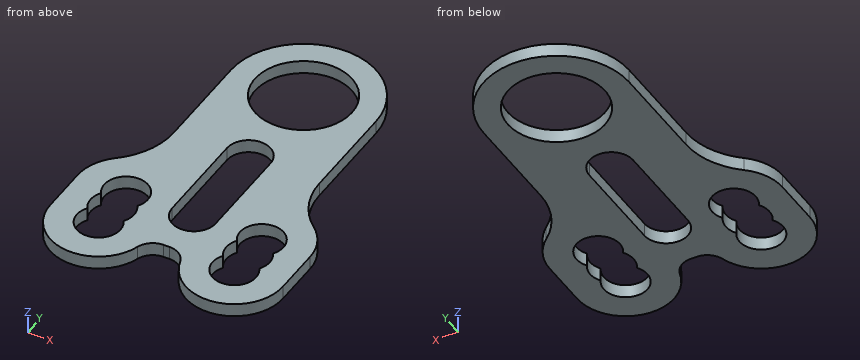
```python
from build123d import *

# Parameters (mm, degrees)
SKETCH_1_R      = 10
EXTRUDE_1_DEPTH = 2.75


with BuildPart() as part:
    # 草图1 → 凸台-拉伸1 (new body)
    with BuildSketch(Plane.XY):
        with BuildLine():
            Line((-24, -40), (-24, -50))
            ThreePointArc((-24, -50), (-15.443695821, -59.895238369), (-4.416851525, -52.857142857))
            ThreePointArc((-4.416851525, -52.857142857), (-2.974049354, -50.792865097), (-0.583592135, -50))
            Line((-0.583592135, -50), (0.583592135, -50))
            ThreePointArc((0.583592135, -50), (2.974049354, -50.792865097), (4.416851525, -52.857142857))
            ThreePointArc((4.416851525, -52.857142857), (15.443695821, -59.895238369), (24, -50))
            Line((24, -50), (24, -40))
            ThreePointArc((24, -40), (23.055385138, -35.757359313), (20.4, -32.316250915))
            ThreePointArc((20.4, -32.316250915), (16.416922293, -27.154588318), (15, -20.790627288))
            Line((15, -20.790627288), (15, 0))
            ThreePointArc((15, 0), (0, 15), (-15, 0))
            Line((-15, 0), (-15, -20.790627288))
            ThreePointArc((-15, -20.790627288), (-16.416922293, -27.154588318), (-20.4, -32.316250915))
            ThreePointArc((-20.4, -32.316250915), (-23.055385138, -35.757359313), (-24, -40))
        make_face()
        Circle(SKETCH_1_R, mode=Mode.SUBTRACT)
        with BuildLine():
            Line((-4.5, -20), (-4.5, -40))
            ThreePointArc((-4.5, -40), (0, -44.5), (4.5, -40))
            Line((4.5, -40), (4.5, -20))
            ThreePointArc((4.5, -20), (0, -15.5), (-4.5, -20))
        make_face(mode=Mode.SUBTRACT)
        with BuildLine():
            ThreePointArc((-17.741657387, -47.5), (-14, -54.5), (-10.258342613, -47.5))
            ThreePointArc((-10.258342613, -47.5), (-9.5, -45), (-10.258342613, -42.5))
            ThreePointArc((-10.258342613, -42.5), (-14, -35.5), (-17.741657387, -42.5))
            ThreePointArc((-17.741657387, -42.5), (-18.5, -45), (-17.741657387, -47.5))
        make_face(mode=Mode.SUBTRACT)
        with BuildLine():
            ThreePointArc((10.258342613, -47.5), (9.5, -45), (10.258342613, -42.5))
            ThreePointArc((10.258342613, -42.5), (14, -35.5), (17.741657387, -42.5))
            ThreePointArc((17.741657387, -42.5), (18.5, -45), (17.741657387, -47.5))
            ThreePointArc((17.741657387, -47.5), (14, -54.5), (10.258342613, -47.5))
        make_face(mode=Mode.SUBTRACT)
    extrude(amount=EXTRUDE_1_DEPTH)


solid = part.part
```
Work out the finished part from the listing and answer in its coordinate system (mm). Give positions to 0.01 mm unless a question says otherwise; leave off trailing zeros. Write each loop counter-clockwise with the first axis right and the second up, starting at its lowest first coordinate (ties: lowest second). Pieces come first, ordered by that corner, then holes. Notation, with made-up numbers: (79, 64) - (89, 64) arc R18 ccw to (89, 81) - close; hole circle Ø5 at (-31.75, 74). An arc over 180 degrees is marked (long way). Use one line per item in the form item = value.
1. A cutting plane is placed at A-A (y = -8). Write down the section's boundary in (x, z).
Filled in:
outline = (-15, 0) - (-6, 0) - (-6, 2.75) - (-15, 2.75) - close; (6, 0) - (15, 0) - (15, 2.75) - (6, 2.75) - close
2. A cutting plane is placed at D-D (y = -46). Write down the section's boundary in (x, z).
Filled in:
outline = (-24, 0) - (-18.39, 0) - (-18.39, 2.75) - (-24, 2.75) - close; (-9.61, 0) - (9.61, 0) - (9.61, 2.75) - (-9.61, 2.75) - close; (18.39, 0) - (24, 0) - (24, 2.75) - (18.39, 2.75) - close
3. Each of these flat-tipped pins is pushed along its axis until it touches: pin 1 Ø1 at (y, z) = (-6.5, 0.5) entering from -X; pin 2 Ø1.4 at (y, z) = (-26.5, 2) entering from -X; pin 3 Ø12 at (x, y) = (2, -34.5) entering from +Z; pin 4 Ø8 at (x, y) = (14, -40) entering from +Z. Where does it stop, or does it pass through?
Filled in:
pin_1 = -15
pin_2 = -16.44
pin_3 = 2.75
pin_4 = through
4. A cutting plane is placed at B-B (z = 1.15). Write down the section's boundary in (x, y), and give its area (3 significant figures).
Filled in:
outline = (-24, -50) arc R10 ccw to (-4.42, -52.86) arc R4 cw to (-0.58, -50) - (0.58, -50) arc R4 cw to (4.42, -52.86) arc R10 ccw to (24, -50) - (24, -40) arc R10 ccw to (20.4, -32.32) arc R15 cw to (15, -20.79) - (15, 0) arc R15 ccw to (-15, 0) - (-15, -20.79) arc R15 cw to (-20.4, -32.32) arc R10 ccw to (-24, -40) - close; hole (-17.74, -47.5) arc R4.5 ccw (long way) to (-10.26, -47.5) arc R4.5 ccw to (-10.26, -42.5) arc R4.5 ccw (long way) to (-17.74, -42.5) arc R4.5 ccw to start; hole circle Ø20 at (0, 0); hole (-4.5, -40) arc R4.5 ccw to (4.5, -40) - (4.5, -20) arc R4.5 ccw to (-4.5, -20) - close; hole (10.26, -47.5) arc R4.5 ccw (long way) to (17.74, -47.5) arc R4.5 ccw to (17.74, -42.5) arc R4.5 ccw (long way) to (10.26, -42.5) arc R4.5 ccw to start
area = 1,660 mm^2
5. A cutting plane is placed at C-C (x = 14). Write down the section's boundary in (y, z).
Filled in:
outline = (-60, 0) - (-54.5, 0) - (-54.5, 2.75) - (-60, 2.75) - close; (-35.5, 0) - (5.39, 0) - (5.39, 2.75) - (-35.5, 2.75) - close
6. Consider L1, parallel to X at y = -40, z = 1.2; L2, parallel to Y at x = 3, z = 1.1; L3, parallel to X at y = -36.5, z = 2.2. Determine where each line is inside the solid, lowest interval first.
Filled in:
L1 = -24 to -18.5, -9.5 to -4.5, 4.5 to 9.5, 18.5 to 24
L2 = -50.81 to -43.35, -16.65 to -9.54, 9.54 to 14.7
L3 = -23.37 to -16.83, -11.17 to -4.5, 4.5 to 11.17, 16.83 to 23.37
